Could you check a few things on this model? Use its own coordinates, in mm. A direction names the side the tool comes from. Coordinates: 2 decimals unless noted, no trailing zeros. Order: outer loops, then holes, each group sorted by start corner. A loop starts at its lowest first (then second) coordinate and runs counter-clockwise, first axis right, second up. Notation, with made-up numbers: (86, 41) - (95, 41) arc R21 cw to (95, 76) - close; hole circle Ø11 at (35, -1). An arc over 180 degrees is marked (long way). Answer as a JSON object with one key per item and string values. Group by question number.
(1) We'd pull the mould along X, two halves only. Please class faces 1 (the flat face through (-47, 42, 3)), 2 (the flat face through (-101, 30, 10)), 3 (the flat face through (0, 30, 5)): pulls with the +X half, pulls with the -X half, needs draft (parallel to the pull), parting line crosses it, or undercut.
(2) Imagine slicing it at C-C, the plane z = 1.5. Write out the boundary of the cut face in (x, y).
(3) Imagine slicing it at B-B, the plane y = 45. Write out the boundary of the cut face in (x, z), and give its area (3 significant figures).
(4) Which directions (+Z, -Z, +X, -X, +Y, -Y) give clear straight access to the entire face, cutting with the end or side of a thin tool? Please do faces 4 (the cylindrical face through (-170.24, 26.35, 3.45)), 5 (the cylindrical face through (-147.043, 15.931, 1.521)), 6 (the cylindrical face through (-154.76, 41.35, 6.55)).
(5) Will these pins go through, and if not, where does the flat tip stop? P1, Ø6, axis at x = -148.5, y = 16, coming from the +Z side; P2, Ø5, axis at x = -50, y = 45, coming from the +Z side.
(6) Please list where these lines run through material, in increasing order: probe 1 along X at (y, z) = (30.5, 4.5); probe 2 along Y at (x, z) = (-150, 1.95); probe 3 along X at (y, z) = (45.5, 8.5).
(7) Imagine slicing it at D-D, the plane x = -175. Write out the boundary of the cut face in (y, z).
(8) Imagine slicing it at A-A, the plane x = -50. Write out the boundary of the cut face in (y, z).
Autodesk Inventor part; units mm, degrees
ref_plane "YZ-Ebene" through (0, 0, 0) normal (1, 0, 0) x (0, 1, 0)
ref_plane "XZ-Ebene" through (0, 0, 0) normal (0, 1, 0) x (-1, 0, 0)
ref_plane "XY-Ebene" through (0, 0, 0) normal (0, 0, 1) x (1, 0, 0)
sketch "Skizze1" plane through (0, 0, 0) normal (0, 0, 1) x (1, 0, 0)
  line L0 (-200, 60) -> (0, 60)
  line L1 (0, 60) -> (0, 0)
  line L2 (0, 0) -> (-200, 0)
  line L3 (-200, 0) -> (-200, 60)
  dimension "d0" = 200
  dimension "d1" = 60
extrude "Extrusion1" add sketch "Skizze1" along normal blind 10
sketch "Skizze2" plane through (0, 0, 10) normal (0, 0, 1) x (1, 0, 0)
  circle A0 centre (-175, 30) radius 3.1
  circle A1 centre (-25, 30) radius 3.1
  line L0 (-200, 0) -> (0, 0)
  line L1 (0, 0) -> (0, 60)
  circle A2 centre (-150, 45) radius 3.1
  circle A3 centre (-50, 45) radius 3.1
  circle A4 centre (-150, 15) radius 3.1
  circle A5 centre (-50, 15) radius 3.1
  line L2 (0, 60) -> (-200, 60)
  dimension "d4" = 6.2
  dimension "d5" = 6.2
  dimension "d6" = 30
  dimension "d7" = 30
  dimension "d8" = 150
  dimension "d9" = 25
  dimension "d10" = 6.2
  dimension "d11" = 6.2
  dimension "d12" = 6.2
  dimension "d13" = 6.2
  dimension "d14" = 30
  dimension "d15" = 30
  dimension "d16" = 100
  dimension "d17" = 100
  dimension "d18" = 50
  dimension "d19" = 50
  dimension "d20" = 15
  dimension "d21" = 15
extrude "Extrusion2" cut sketch "Skizze2" against normal blind 15
sketch "Skizze3" plane through (0, 0, 10) normal (0, 0, 1) x (1, 0, 0)
  circle A0 centre (-150, 45) radius 3.1
  circle A1 centre (-150, 45) radius 6
  circle A2 centre (-150, 15) radius 3.1
  circle A3 centre (-150, 15) radius 6
  circle A4 centre (-50, 45) radius 3.1
  circle A5 centre (-50, 15) radius 3.1
  circle A6 centre (-50, 15) radius 6
  circle A7 centre (-50, 45) radius 6
  point P0 (0, 0)
  dimension "d24" = 12
  dimension "d25" = 12
  dimension "d26" = 12
  dimension "d27" = 12
extrude "Extrusion3" cut sketch "Skizze3" against normal blind 7 contours A1 | A3 | A5 | A6 | A7
sketch "Skizze4" plane through (0, 0, 0) normal (0, 0, -1) x (-1, 0, 0)
  circle A0 centre (175, 30) radius 3.1
  circle A1 centre (175, 30) radius 6
  circle A2 centre (25, 30) radius 3.1
  circle A3 centre (25, 30) radius 6
  point P0 (0, 0)
  dimension "d30" = 12
  dimension "d31" = 12
extrude "Extrusion4" cut sketch "Skizze4" against normal blind 7 contours A0 | A1 | A2 | A3
properties part number "adapter_stage"
Result set:
{
 "1": {"face 1": "undercut", "face 2": "needs draft", "face 3": "pulls with the +X half"},
 "2": {"outline": "(-200, 0) - (0, 0) - (0, 60) - (-200, 60) - close; hole circle Ø12 at (-175, 30); hole circle Ø6.2 at (-150, 15); hole circle Ø6.2 at (-150, 45); hole circle Ø6.2 at (-50, 15); hole circle Ø6.2 at (-50, 45); hole circle Ø12 at (-25, 30)"},
 "3": {"outline": "(-200, 0) - (-153.1, 0) - (-153.1, 3) - (-156, 3) - (-156, 10) - (-200, 10) - close; (-146.9, 0) - (-53.1, 0) - (-53.1, 3) - (-56, 3) - (-56, 10) - (-144, 10) - (-144, 3) - (-146.9, 3) - close; (-46.9, 0) - (0, 0) - (0, 10) - (-44, 10) - (-44, 3) - (-46.9, 3) - close", "area": "1,790 mm^2"},
 "4": {"face 4": "-Z", "face 5": "+Z, -Z", "face 6": "+Z"},
 "5": {"P1": "stops at z = 3", "P2": "passes through"},
 "6": {"probe 1": "x = -200 to -180.98, -169.02 to -30.98, -19.02 to 0", "probe 2": "y = 0 to 11.9, 18.1 to 41.9, 48.1 to 60", "probe 3": "x = -200 to -155.98, -144.02 to -55.98, -44.02 to 0"},
 "7": {"outline": "(0, 0) - (24, 0) - (24, 7) - (26.9, 7) - (26.9, 10) - (0, 10) - close; (33.1, 7) - (36, 7) - (36, 0) - (60, 0) - (60, 10) - (33.1, 10) - close"},
 "8": {"outline": "(0, 0) - (11.9, 0) - (11.9, 3) - (9, 3) - (9, 10) - (0, 10) - close; (18.1, 0) - (41.9, 0) - (41.9, 3) - (39, 3) - (39, 10) - (21, 10) - (21, 3) - (18.1, 3) - close; (48.1, 0) - (60, 0) - (60, 10) - (51, 10) - (51, 3) - (48.1, 3) - close"}
}
